Can you work these out from the model? Positions are in its coordinate system, mm. A direction names the side the tool comes from. Give positions to 0.01 mm unless a question says otherwise; leave off trailing zeros. Order: outer loops, then holes, each group sorted by start corner. A loop starts at its lowest first (then second) coordinate and runs counter-clockwise, first axis right, second up.
```python
from build123d import *

# Parameters (mm, degrees)
SKETCH1_W           = 137.5
SKETCH1_H           = 98
BOSS_EXTRUDE1_DEPTH = 1.5
SKETCH2_R           = 34
SKETCH2_W           = 107.5
SKETCH2_H           = 47.5
CUT_EXTRUDE1_DEPTH  = 85.478177656
CUT_EXTRUDE3_DEPTH  = 85.478177656
FILLET1_R           = 0.5
SKETCH22_W          = 4.5
SKETCH22_H          = 4
CUT_EXTRUDE5_DEPTH  = 85.478177656
CHAMFER1_SIZE       = 10
CHAMFER2_SIZE       = 2.5


with BuildPart() as part:
    # Sketch1 → Boss-Extrude1 (new, symmetric)
    with BuildSketch(Plane.XY):
        Rectangle(SKETCH1_W, SKETCH1_H)
    extrude(amount=BOSS_EXTRUDE1_DEPTH, both=True)

    # Sketch2 → Cut-Extrude1 (cut, through all)
    with BuildSketch(Plane.XY.offset(1.5)):
        with Locations((1.75, 49)):
            Circle(SKETCH2_R)
        with Locations((0, -25.25)):
            Rectangle(SKETCH2_W, SKETCH2_H)
    extrude(amount=-CUT_EXTRUDE1_DEPTH, mode=Mode.SUBTRACT)

    # Sketch17 → Cut-Extrude3 (cut, through all)
    with BuildSketch(Plane.XY.offset(1.5)):
        with BuildLine():
            Line((1.75, 12.5), (-1.25, 14.630682288))
            ThreePointArc((-1.25, 14.630682288), (-4.98061611, 15.162907826), (-8.630929873, 16.098840522))
            Line((-8.630929873, 16.098840522), (-12.217945281, 15.278397063))
            Line((-12.217945281, 15.278397063), (-14.174207068, 18.394941116))
            ThreePointArc((-14.174207068, 18.394941116), (-17.417173039, 20.314298376), (-20.431457275, 22.575902037))
            Line((-20.431457275, 22.575902037), (-24.059397513, 23.190602487))
            Line((-24.059397513, 23.190602487), (-24.674097963, 26.818542725))
            ThreePointArc((-24.674097963, 26.818542725), (-26.935701624, 29.832826961), (-28.855058884, 33.075792932))
            Line((-28.855058884, 33.075792932), (-31.971602937, 35.032054719))
            Line((-31.971602937, 35.032054719), (-31.151159478, 38.619070127))
            ThreePointArc((-31.151159478, 38.619070127), (1.75, 83.5), (34.651159478, 38.619070127))
            Line((34.651159478, 38.619070127), (35.471602937, 35.032054719))
            Line((35.471602937, 35.032054719), (32.355058884, 33.075792932))
            ThreePointArc((32.355058884, 33.075792932), (30.435701624, 29.832826961), (28.174097963, 26.818542725))
            Line((28.174097963, 26.818542725), (27.559397513, 23.190602487))
            Line((27.559397513, 23.190602487), (23.931457275, 22.575902037))
            ThreePointArc((23.931457275, 22.575902037), (20.917173039, 20.314298376), (17.674207068, 18.394941116))
            Line((17.674207068, 18.394941116), (15.717945281, 15.278397063))
            Line((15.717945281, 15.278397063), (12.130929873, 16.098840522))
            ThreePointArc((12.130929873, 16.098840522), (8.48061611, 15.162907826), (4.75, 14.630682288))
            Line((4.75, 14.630682288), (1.75, 12.5))
        make_face()
    extrude(amount=-CUT_EXTRUDE3_DEPTH, mode=Mode.SUBTRACT)

    # Fillet1
    fillet1_edges = [part.edges().sort_by_distance(p)[0] for p in [
        (15.717945281, 15.278397063, 0),
        (1.75, 12.5, 0),
        (-12.217945281, 15.278397063, 0),
        (-24.059397513, 23.190602487, 0),
        (-31.971602937, 35.032054719, 0),
        (35.471602937, 35.032054719, 0),
        (27.559397513, 23.190602487, 0),
    ]]
    fillet(fillet1_edges, radius=FILLET1_R)

    # Sketch22 → Cut-Extrude5 (cut, through all)
    with BuildSketch(Plane(origin=(0, 0, -1.5), x_dir=(-1, 0, 0), z_dir=(0, 0, -1))):
        with Locations((-66.5, -47)):
            Rectangle(SKETCH22_W, SKETCH22_H)
        with Locations((66.5, -47)):
            Rectangle(SKETCH22_W, SKETCH22_H)
        with Locations((56, -47)):
            Rectangle(SKETCH22_W, SKETCH22_H)
        with Locations((-56, -47)):
            Rectangle(SKETCH22_W, SKETCH22_H)
    extrude(amount=-CUT_EXTRUDE5_DEPTH, mode=Mode.SUBTRACT)

    # Chamfer1
    chamfer1_edges = [part.edges().sort_by_distance(p)[0] for p in [
        (-53.75, -1.5, 0),
        (53.75, -1.5, 0),
        (-68.75, 49, 0),
        (68.75, 49, 0),
    ]]
    chamfer(chamfer1_edges, length=CHAMFER1_SIZE)

    # Chamfer2
    # the kernel refuses this chamfer: 2.5 mm, written as the material it takes off along each edge
    with BuildSketch(Plane(origin=(36.25, 49, -8.184978913), x_dir=(1, 0, 0), z_dir=(0, 0, 1))) as chamfer2_piece_1:
        with BuildLine():
            Line((CHAMFER2_SIZE, 0), (-0.097956106, -2.597956106))
            ThreePointArc((-0.097956106, -2.597956106), (-0.025900977, -1.336598881), (0, 0))
            Line((0, 0), (CHAMFER2_SIZE, 0))
        make_face()
    extrude(amount=16.369957825, mode=Mode.SUBTRACT)
    with BuildSketch(Plane(origin=(-32.75, 49, -8.184978913), x_dir=(-1, 0, 0), z_dir=(0, 0, 1))) as chamfer2_piece_2:
        with BuildLine():
            Line((CHAMFER2_SIZE, 0), (-0.097956106, 2.597956106))
            ThreePointArc((-0.097956106, 2.597956106), (-0.025900977, 1.336598881), (0, 0))
            Line((0, 0), (CHAMFER2_SIZE, 0))
        make_face()
    extrude(amount=16.369957825, mode=Mode.SUBTRACT)


solid = part.part
```
1) If I drill on line 1 (X direction, y = -37, z = -1.25); line 2 (Y direction, x = 5, z = -0.25); line 3 (Y direction, x = -18, z = 0.9), over which ranges is the centre line in solid material (lowest first)?
2) Suppose I cut it at A-A (y = -38). Please give me the cut outline in (x, z), and give its area (3 significant figures).
3) We'd pull the mould along X, two halves only. Please class faces 4 (the face through (63.82, 43.93, 0.02)), 5 (the face through (67, -45, 0)), 6 (the face through (8.532, 15.173, 0.021)): +X half, -X half, draft (parallel to the pull), parting line (faces both ways), or undercut.
4) I'm going to push flat-ended pins straight in: pin 1 Ø1.5 at (y, z) = (-47.5, -0.5) entering from -X; pin 2 Ø0.9 at (x, z) = (-67, -0.5) entering from -Y; pin 3 Ø1.5 at (y, z) = (-46.5, -0.5) entering from +X. Where does each tip first touch, or does it pass through?
5) Suppose I cut it at C-C (x = -10). Please give me the cut outline in (y, z), and give its area (3 significant figures).
6) Suppose I cut it at B-B (x = -38.5). Please give me the cut outline in (y, z).
7) Which directions (+Z, -Z, +X, -X, +Y, -Y) give clear straight access to the entire face, cutting with the end or side of a thin tool? Please do faces 1 (the face through (-30.243, 33.947, 0.021)), 2 (the face through (56, -45, 0)), 3 (the face through (-10.229, 15.733, 0.021)).
Results:
1. line 1: x = -68.75 to -53.75, 53.75 to 68.75
1. line 2: y = -1.5 to 14.65
1. line 3: y = -1.5 to 20.71
2. outline: (-68.75, -1.5) - (-53.75, -1.5) - (-53.75, 1.5) - (-68.75, 1.5) - close; (53.75, -1.5) - (68.75, -1.5) - (68.75, 1.5) - (53.75, 1.5) - close
2. area: 90.0 mm2
3. face 4: +X half
3. face 5: draft
3. face 6: undercut
4. pin 1: stops at x = -64.25
4. pin 2: stops at y = -45
4. pin 3: stops at x = 64.25
5. outline: (-1.5, -1.5) - (15.79, -1.5) - (15.79, 1.5) - (-1.5, 1.5) - close
5. area: 51.9 mm2
6. outline: (-1.5, -1.5) - (49, -1.5) - (49, 1.5) - (-1.5, 1.5) - close
7. face 1: +Z, -Z
7. face 2: +Z, -Z, -Y
7. face 3: +Z, -Z, +Y
